Work out the finished part from the listing and answer in its coordinate system (mm). Face numbers are marked on the shaded views. A direction names the side the tool comes from. Round coordinates to 2 decimals unless told otherwise and drop trailing zeros. Order: outer loops, then holes, each group sorted by start corner. A loop starts at its lowest first (then second) coordinate and runs counter-clockwise, first axis right, second up. Notation, with made-up numbers: (87, -11.75) -> (105, -11.75) arc R19 cw to (105, -2.75) -> close; hole circle Ø4 at (-32, 43). An arc over 180 degrees is marked (long way). Use one line per item in the form item = value.
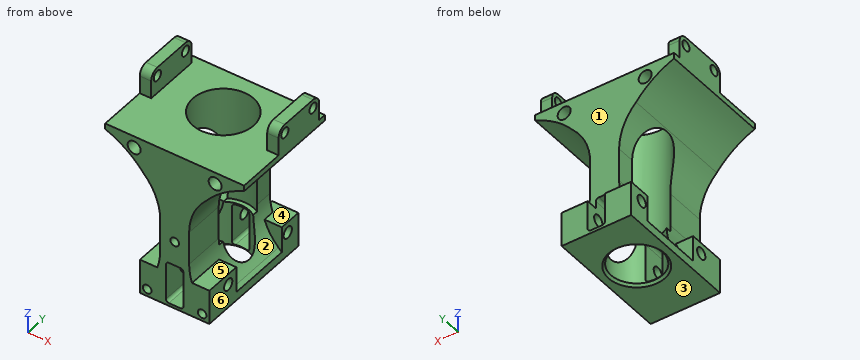
```python
from build123d import *

# Parameters (mm, degrees)
SKETCH_1_W                = 48
SKETCH_1_H                = 31
SKETCH_1_R                = 8.9
EXTRUDE_1_DEPTH           = 65
SKETCH_2_R                = 10.5
CUT_EXTRUDE_1_DEPTH       = 49
CUT_EXTRUDE_3_DEPTH       = 76.907838857
CUT_EXTRUDE_START         = -31
CUT_EXTRUDE_5_DEPTH       = 107.907838984
SKETCH_9_R                = 1.5
CUT_EXTRUDE_6_DEPTH       = 7
CUT_EXTRUDE_START_2       = -24
SKETCH_9_2_R              = 1.5
CUT_EXTRUDE_7_DEPTH       = 7
EXTRUDE_4_DEPTH           = 8
SKETCH_11_R               = 2.25
CUT_EXTRUDE_9_DEPTH       = 80.511005658
SKETCH_14_R               = 1.5
CUT_EXTRUDE_10_DEPTH      = 11
SKETCH_15_W               = 40.1
SKETCH_15_H               = 9.5
CUT_EXTRUDE_11_DEPTH      = 80.511005658
SKETCH_17_R               = 1.75
CUT_EXTRUDE_13_DEPTH      = 85.150163426
SKETCH_19_W               = 3
SKETCH_19_H               = 3
CUT_EXTRUDE_14_DEPTH      = 76.651107105
CHAMFER_1_SIZE            = 0.8
EXTRUDE_START             = 8
SKETCH_21_R               = 1.5
EXTRUDE_6_DEPTH           = 8
EXTRUDE_START_2           = -13
EXTRUDE_7_DEPTH           = 13
EXTRUDE_8_DEPTH           = 4
EXTRUDE_8_DEPTH_BACK      = 4
CUT_EXTRUDE_15_DEPTH      = 73.899519921
CUT_EXTRUDE_15_DEPTH_BACK = 73.899519921
SKETCH_20_R               = 2


with BuildPart() as part:
    # 草图1 → 凸台-拉伸1 (new body)
    with BuildSketch(Plane.XY):
        Rectangle(SKETCH_1_W, SKETCH_1_H)
        Circle(SKETCH_1_R, mode=Mode.SUBTRACT)
    extrude(amount=EXTRUDE_1_DEPTH)

    # 草图2 → 切除-拉伸1 (cut)
    with BuildSketch(Plane.XY.offset(65)):
        Circle(SKETCH_2_R)
    extrude(amount=-CUT_EXTRUDE_1_DEPTH, mode=Mode.SUBTRACT)

    # 草图4 → 切除-拉伸3 (cut, through all)
    with BuildSketch(Plane(origin=(0, 15.5, 0), x_dir=(1, 0, 0), z_dir=(0, 1, 0))):
        with BuildLine():
            Line((-24, 9), (-10.857864376, -4.142135624))
            ThreePointArc((-10.857864376, -4.142135624), (-6.52240935, -10.6306026), (-5, -18.284271247))
            Line((-5, -18.284271247), (-5, -29.715728753))
            ThreePointArc((-5, -29.715728753), (-6.52240935, -37.3693974), (-10.857864376, -43.857864376))
            ThreePointArc((-10.857864376, -43.857864376), (-16.798925034, -49.531146093), (-24, -53.484226727))
            Line((-24, -53.484226727), (-24, 9))
        make_face()
        with BuildLine():
            Line((5, -18.284271247), (5, -29.715728753))
            ThreePointArc((5, -29.715728753), (6.52240935, -37.3693974), (10.857864376, -43.857864376))
            ThreePointArc((10.857864376, -43.857864376), (16.798925034, -49.531146093), (24, -53.484226727))
            Line((24, -53.484226727), (24, 9))
            Line((24, 9), (10.857864376, -4.142135624))
            ThreePointArc((10.857864376, -4.142135624), (6.52240935, -10.6306026), (5, -18.284271247))
        make_face()
    extrude(amount=-CUT_EXTRUDE_3_DEPTH, mode=Mode.SUBTRACT)

    # 草图6 → 切除-拉伸5 (cut, through all)
    with BuildSketch(Plane(origin=(0, 15.5, 0), x_dir=(1, 0, 0), z_dir=(0, 1, 0)).offset(CUT_EXTRUDE_START)):
        with BuildLine():
            Line((-2, -1), (2, -1))
            ThreePointArc((2, -1), (2.707106781, -1.292893219), (3, -2))
            Line((3, -2), (3, -14.5))
            ThreePointArc((3, -14.5), (2.707106781, -15.207106781), (2, -15.5))
            Line((2, -15.5), (-2, -15.5))
            ThreePointArc((-2, -15.5), (-2.707106781, -15.207106781), (-3, -14.5))
            Line((-3, -14.5), (-3, -2))
            ThreePointArc((-3, -2), (-2.707106781, -1.292893219), (-2, -1))
        make_face()
    extrude(amount=CUT_EXTRUDE_5_DEPTH, mode=Mode.SUBTRACT)

    # 草图9 → 切除-拉伸6 (cut)
    with BuildSketch(Plane(origin=(0, 15.5, 0), x_dir=(1, 0, 0), z_dir=(0, 1, 0))):
        with Locations(Location((9.5, -2.5, 0), (0, 0, 270))):
            Circle(SKETCH_9_R)
        with Locations(Location((-9.5, -2.5, 0), (0, 0, 270))):
            Circle(SKETCH_9_R)
    extrude(amount=-CUT_EXTRUDE_6_DEPTH, mode=Mode.SUBTRACT)

    # 草图9<2> → 切除-拉伸7 (cut)
    with BuildSketch(Plane(origin=(0, 15.5, 0), x_dir=(1, 0, 0), z_dir=(0, 1, 0)).offset(CUT_EXTRUDE_START_2)):
        with Locations(Location((9.5, -2.5, 0), (0, 0, 270))):
            Circle(SKETCH_9_2_R)
        with Locations(Location((-9.5, -2.5, 0), (0, 0, 270))):
            Circle(SKETCH_9_2_R)
    extrude(amount=-CUT_EXTRUDE_7_DEPTH, mode=Mode.SUBTRACT)

    # 草图12 → 凸台-拉伸4 (add)
    with BuildSketch(Plane.XZ.offset(15.5)):
        with BuildLine():
            Line((-5, 18.284271247), (5, 18.284271247))
            Line((5, 18.284271247), (5, 29.715728753))
            ThreePointArc((5, 29.715728753), (6.52240935, 37.3693974), (10.857864376, 43.857864376))
            ThreePointArc((10.857864376, 43.857864376), (16.798925034, 49.531146093), (24, 53.484226727))
            Line((24, 53.484226727), (24, 65))
            Line((24, 65), (-24, 65))
            Line((-24, 65), (-24, 53.484226727))
            ThreePointArc((-24, 53.484226727), (-16.798925034, 49.531146093), (-10.857864376, 43.857864376))
            ThreePointArc((-10.857864376, 43.857864376), (-6.52240935, 37.3693974), (-5, 29.715728753))
            Line((-5, 29.715728753), (-5, 18.284271247))
        make_face()
    extrude(amount=EXTRUDE_4_DEPTH)

    # 草图11 → 切除-拉伸9 (cut, through all)
    with BuildSketch(Plane(origin=(0, 15.5, 0), x_dir=(1, 0, 0), z_dir=(0, 1, 0))):
        with Locations(Location((14, -51.5, 0), (0, 0, 270))):
            Circle(SKETCH_11_R)
        with Locations(Location((-14, -51.5, 0), (0, 0, 270))):
            Circle(SKETCH_11_R)
    extrude(amount=-CUT_EXTRUDE_9_DEPTH, mode=Mode.SUBTRACT)

    # 草图14 → 切除-拉伸10 (cut)
    with BuildSketch(Plane.XZ.offset(23.5)):
        with Locations(Location((0, 24, 0), (0, 0, 270))):
            Circle(SKETCH_14_R)
    extrude(amount=-CUT_EXTRUDE_10_DEPTH, mode=Mode.SUBTRACT)

    # 草图15 → 切除-拉伸11 (cut, through all)
    with BuildSketch(Plane(origin=(0, 15.5, 0), x_dir=(1, 0, 0), z_dir=(0, 1, 0))):
        with Locations((0, -60.25)):
            Rectangle(SKETCH_15_W, SKETCH_15_H)
    extrude(amount=-CUT_EXTRUDE_11_DEPTH, mode=Mode.SUBTRACT)

    # 草图17 → 切除-拉伸13 (cut, through all)
    with BuildSketch(Plane(origin=(24, 0, 0), x_dir=(0, 0, -1), z_dir=(1, 0, 0))):
        with Locations((-61.7, 9.8)):
            Circle(SKETCH_17_R)
        with Locations((-61.7, -3.8)):
            Circle(SKETCH_17_R)
        with BuildLine():
            Line((-55.5, -23.5), (-55.5, -6.8))
            Line((-55.5, -6.8), (-61.7, -6.8))
            ThreePointArc((-61.7, -6.8), (-63.821320344, -5.921320344), (-64.7, -3.8))
            Line((-64.7, -3.8), (-64.7, 9.8))
            ThreePointArc((-64.7, 9.8), (-63.821320344, 11.921320344), (-61.7, 12.8))
            Line((-61.7, 12.8), (-55.5, 12.8))
            Line((-55.5, 12.8), (-55.5, 15.5))
            Line((-55.5, 15.5), (-64.7, 15.5))
            Line((-64.7, 15.5), (-94.5, 15.5))
            Line((-94.5, 15.5), (-94.5, -23.5))
            Line((-94.5, -23.5), (-55.5, -23.5))
        make_face()
    extrude(amount=-CUT_EXTRUDE_13_DEPTH, mode=Mode.SUBTRACT)

    # 草图19 → 切除-拉伸14 (cut, through all)
    with BuildSketch(Plane.XZ.offset(15.5)):
        with Locations((-13.5, 1.5)):
            Rectangle(SKETCH_19_W, SKETCH_19_H)
        with Locations((13.5, 1.5)):
            Rectangle(SKETCH_19_W, SKETCH_19_H)
    extrude(amount=-CUT_EXTRUDE_14_DEPTH, mode=Mode.SUBTRACT)

    # 倒角1
    chamfer_1_edges = [part.edges().sort_by_distance(p)[0] for p in [
        (-8.9, 0, 0),
    ]]
    chamfer(chamfer_1_edges, length=CHAMFER_1_SIZE)

    # 草图21 → 凸台-拉伸6 (add)
    with BuildSketch(Plane.XZ.offset(15.5).offset(EXTRUDE_START)):
        with BuildLine():
            Line((-10.857864376, 4.142135624), (-12, 3))
            Line((-12, 3), (-12, 0))
            Line((-12, 0), (12, 0))
            Line((12, 0), (12, 3))
            Line((12, 3), (10.857864376, 4.142135624))
            ThreePointArc((10.857864376, 4.142135624), (6.52240935, 10.6306026), (5, 18.284271247))
            Line((5, 18.284271247), (-5, 18.284271247))
            ThreePointArc((-5, 18.284271247), (-6.52240935, 10.6306026), (-10.857864376, 4.142135624))
        make_face()
        with Locations(Location((9.5, 2.5, 0), (0, 0, 90))):
            Circle(SKETCH_21_R, mode=Mode.SUBTRACT)
        with Locations(Location((-9.5, 2.5, 0), (0, 0, 90))):
            Circle(SKETCH_21_R, mode=Mode.SUBTRACT)
        with BuildLine():
            Line((2, 1), (-2, 1))
            ThreePointArc((-2, 1), (-2.707106781, 1.292893219), (-3, 2))
            Line((-3, 2), (-3, 14.5))
            ThreePointArc((-3, 14.5), (-2.707106781, 15.207106781), (-2, 15.5))
            Line((-2, 15.5), (2, 15.5))
            ThreePointArc((2, 15.5), (2.707106781, 15.207106781), (3, 14.5))
            Line((3, 14.5), (3, 2))
            ThreePointArc((3, 2), (2.707106781, 1.292893219), (2, 1))
        make_face(mode=Mode.SUBTRACT)
    extrude(amount=-EXTRUDE_6_DEPTH)

    # 草图22 → 凸台-拉伸7 (add)
    with BuildSketch(Plane.XZ.offset(23.5).offset(EXTRUDE_START_2)):
        with BuildLine():
            Line((12, 3), (12, 12))
            Line((12, 12), (6.012953497, 12))
            ThreePointArc((6.012953497, 12), (7.975835256, 7.787709202), (10.857864376, 4.142135624))
            Line((10.857864376, 4.142135624), (12, 3))
        make_face()
    extrude_7 = extrude(amount=EXTRUDE_7_DEPTH)

    # 镜向1: 凸台-拉伸7 across plane
    add(extrude_7.mirror(Plane(origin=(0, 0, 0), x_dir=(0, 0, 1), z_dir=(1, 0, 0))))

    # 草图23 → 凸台-拉伸8 (add, two sides: drawn at the far end of the back side and taken through both)
    with BuildSketch(Plane(origin=(0, 15.5, 0), x_dir=(1, 0, 0), z_dir=(0, 1, 0)).offset(-EXTRUDE_8_DEPTH_BACK)):
        with BuildLine():
            Line((-12, 0), (-12, -12))
            Line((-12, -12), (-3, -12))
            Line((-3, -12), (-3, -2))
            ThreePointArc((-3, -2), (-2.707106781, -1.292893219), (-2, -1))
            Line((-2, -1), (2, -1))
            ThreePointArc((2, -1), (2.707106781, -1.292893219), (3, -2))
            Line((3, -2), (3, -12))
            Line((3, -12), (6.012953497, -12))
            Line((6.012953497, -12), (12, -12))
            Line((12, -12), (12, 0))
            Line((12, 0), (-12, 0))
        make_face()
    extrude(amount=EXTRUDE_8_DEPTH + EXTRUDE_8_DEPTH_BACK)

    # 草图20 → 切除-拉伸15 (cut, two sides: drawn at the far end of the back side and taken through both)
    with BuildSketch(Plane(origin=(0, 0, 0), x_dir=(0, 0, -1), z_dir=(1, 0, 0)).offset(-CUT_EXTRUDE_15_DEPTH_BACK)):
        with Locations(Location((-8.25, 14.4, 0), (0, 0, 180))):
            Circle(SKETCH_20_R)
        with Locations(Location((-8.25, -14.4, 0), (0, 0, 180))):
            Circle(SKETCH_20_R)
    extrude(amount=CUT_EXTRUDE_15_DEPTH + CUT_EXTRUDE_15_DEPTH_BACK, mode=Mode.SUBTRACT)


solid = part.part
```
Item 1: Flat-ended cylindrical pins translate along their axes: P1, Ø12, axis at y = -10.5, z = 13.5, coming from the -X side; P2, Ø3, axis at x = -17, y = -18.5, coming from the +Z side; P3, Ø3, axis at y = 14.4, z = 8.25, coming from the +X side; P4, Ø4.5, axis at y = 14.4, z = 8.25, coming from the +X side. Find the tip coordinate at first contact, or state that the pin passes through.
Findings:
P1 = -12
P2 = 55.5
P3 = through
P4 = 12
Item 2: The part is cut by section C-C, the plane z = 52. Give the vertices of the cut face in (x, y).
Findings:
outline = (-20.75, -23.5) -> (-16.19, -23.5) -> (-16.19, 15.5) -> (-20.75, 15.5) -> close; (-11.81, -23.5) -> (11.81, -23.5) -> (11.81, 15.5) -> (-11.81, 15.5) -> close; (16.19, -23.5) -> (20.75, -23.5) -> (20.75, 15.5) -> (16.19, 15.5) -> close; hole circle Ø21 at (0, 0)
Item 3: The part is cut by section A-A, the plane y = 14.4. Give the number of separate pieces and of enclosed holes in the cut face, and give its area (3 significant figures).
Findings:
separate_pieces = 2
enclosed_holes = 2
area = 881 mm^2
Item 4: The part is cut by section D-D, the plane z = 24. Give the vertices of the cut face in (x, y), and give its area (3 significant figures).
Findings:
outline = (-5, -23.5) -> (-1.5, -23.5) -> (-1.5, -12.5) -> (1.5, -12.5) -> (1.5, -23.5) -> (5, -23.5) -> (5, -9.23) arc R10.5 cw to (-5, -9.23) -> close; (-5, 9.23) arc R10.5 cw to (5, 9.23) -> (5, 15.5) -> (-5, 15.5) -> close
area = 155 mm^2
Item 5: The part is cut by section B-B, the plane x = 0. Give the vertices of the cut face in (y, z), and give its area (3 significant figures).
Findings:
outline = (-23.5, 0) -> (-9.7, 0) -> (-8.9, 0.8) -> (-8.9, 1) -> (-23.5, 1) -> close; (-23.5, 15.5) -> (-8.9, 15.5) -> (-8.9, 16) -> (-10.5, 16) -> (-10.5, 55.5) -> (-23.5, 55.5) -> (-23.5, 25.5) -> (-12.5, 25.5) -> (-12.5, 22.5) -> (-23.5, 22.5) -> close; (8.9, 0.8) -> (9.7, 0) -> (19.5, 0) -> (19.5, 1) -> (8.9, 1) -> close; (8.9, 15.5) -> (15.5, 15.5) -> (15.5, 55.5) -> (10.5, 55.5) -> (10.5, 16) -> (8.9, 16) -> close
area = 713 mm^2
Item 6: Determine the mould class of the marked faces 1, 2 and 3 for opening direction Z: released by +Z, released by -Z, zero draft, split by the parting line, or undercut.
Findings:
face_1 = zero draft
face_2 = undercut
face_3 = released by -Z
Item 7: For the marked faces 4, 5 and 6, determine the directions among +Z, -Z, +X, -X, +Y, -Y from which every point of the face is accessible in a straight line to the end or side of a thin tool.
Findings:
face_4 = +X, +Y
face_5 = +X, +Y, -Y
face_6 = -Z, +X, +Y, -Y
Item 8: Consider line 1 along X through (y, z) = (10.6, 2.5); line 2 along Y through (x, z) = (8, 8.25); line 3 along Z through (x, y) = (1, 11). Determine where each line is inside the solid, lowest interval first.
Findings:
line_1 = -12 to -11, -8 to -3, 3 to 8, 11 to 12
line_2 = -23.5 to -16.4, -12.4 to -10.5, 11.5 to 12.4, 16.4 to 19.5
line_3 = 0 to 1, 15.5 to 55.5
